Check sheet for the modelled part. Datum: model origin and axes. Units: mm. A direction names the side the tool comes from. Round coordinates to 2 decimals unless told otherwise and drop trailing zeros. Loops run counter-clockwise (first coordinate to the right, second up) from the corner with the lowest first, then second, coordinate; pieces in that order, holes last. Notation, with made-up numbers: (-27, 29) -> (6, 29) arc R31 ccw to (6, 65) -> close; hole circle Ø6 at (-38, 41). An arc over 180 degrees is marked (long way). Return JSON: item names as keys, results as strings.
from build123d import *

# Parameters (mm, degrees)
ESQUISSE1_R        = 0.85
BOSS_EXTRU_1_DEPTH = 0.4


with BuildPart() as part:
    # Esquisse1 → Boss.-Extru.1 (new body)
    with BuildSketch(Plane.XY):
        with BuildLine():
            ThreePointArc((13.321737348, 14.240130408), (-14.376908068, -13.174009049), (15.347008325, 12.029934973))
            ThreePointArc((15.347008325, 12.029934973), (13.270992063, 12.160623737), (13.321737348, 14.240130408))
        make_face()
        Circle(ESQUISSE1_R, mode=Mode.SUBTRACT)
        with BuildLine():
            Line((-14.2, -2.5), (-14.2, 2.5))
            ThreePointArc((-14.2, 2.5), (-11.45, 5.25), (-8.7, 2.5))
            Line((-8.7, 2.5), (-8.7, -2.5))
            ThreePointArc((-8.7, -2.5), (-11.45, -5.25), (-14.2, -2.5))
        make_face(mode=Mode.SUBTRACT)
    extrude(amount=BOSS_EXTRU_1_DEPTH)


solid = part.part
Q1. Section check D-D (y = 7.5). Record the boundary of the cut face in (x, z), then the cut area to 3 significant figures.
Results list:
{"outline": "(-18, 0) -> (18, 0) -> (18, 0.4) -> (-18, 0.4) -> close", "area": "14.4 mm^2"}
Q2. Section check C-C (z = 0.2). Record the boundary of the cut face in (x, y), then the cut area to 3 significant figures.
Results list:
{"outline": "(13.32, 14.24) arc R19.5 ccw (long way) to (15.35, 12.03) arc R1.5 cw to start; hole (-14.2, -2.5) arc R2.75 ccw to (-8.7, -2.5) -> (-8.7, 2.5) arc R2.75 ccw to (-14.2, 2.5) -> close; hole circle Ø1.7 at (0, 0)", "area": "1,140 mm^2"}
Q3. Section check B-B (x = -13). Record the boundary of the cut face in (y, z), then the cut area to 3 significant figures.
Results list:
{"outline": "(-14.53, 0) -> (-4.77, 0) -> (-4.77, 0.4) -> (-14.53, 0.4) -> close; (4.77, 0) -> (14.53, 0) -> (14.53, 0.4) -> (4.77, 0.4) -> close", "area": "7.81 mm^2"}
Q4. Material ranges on line 1 (Y direction, x = 0, z = 0.1); line 2 (X direction, y = -1, z = 0.3); line 3 (Y direction, x = 14, z = 0.15), recorded low to high.
Results list:
{"line 1": "-19.5 to -0.85, 0.85 to 19.5", "line 2": "-19.47 to -14.2, -8.7 to 19.47", "line 3": "-13.57 to 11.72"}
Q5. Section check A-A (y = 0). Record the boundary of the cut face in (x, z).
Results list:
{"outline": "(-19.5, 0) -> (-14.2, 0) -> (-14.2, 0.4) -> (-19.5, 0.4) -> close; (-8.7, 0) -> (-0.85, 0) -> (-0.85, 0.4) -> (-8.7, 0.4) -> close; (0.85, 0) -> (19.5, 0) -> (19.5, 0.4) -> (0.85, 0.4) -> close"}
Q6. Tool access check on faces 1 (the flat face through (4, 0, 0)), 2 (the cylindrical face through (-11.51, 5.25, 0.2)). Record the directions out of +Z, -Z, +X, -X, +Y, -Y that give a thin tool (end or side, any length) a straight path to the whole face; none if there is none.
Results list:
{"face 1": "-Z, +X, -X, +Y, -Y", "face 2": "+Z, -Z"}
Q7. Draft check along X on faces 3 (the cylindrical face through (-11.39, -5.25, 0.2)), 4 (the flat face through (4, 0, 0.4)), 5 (the cylindrical face through (-14.929, -12.545, 0.197)). Enter one of: released by +X, released by -X, zero draft, split by the parting line, or undercut.
Results list:
{"face 3": "undercut", "face 4": "zero draft", "face 5": "split by the parting line"}
